Can you work these out from the model? Positions are in its coordinate system, mm. Face numbers are marked on the shaded views. A direction names the side the tool comes from. Coordinates: 2 decimals unless noted, no trailing zeros. Order: outer loops, then holes, each group sorted by start corner. A loop starts at its lowest first (then second) coordinate and runs counter-clockwise, first axis right, second up. Notation, with made-up numbers: (-35.75, 19) - (22.25, 19) arc R19 cw to (22.25, 55) - close; hole circle Ø2 at (-36, 30). An arc over 180 degrees is marked (long way). Use a Markdown table: item, result. Add a question column.
(1) I want a section at D-D (x = -130). List the corners of the cut face in (y, z) for me.
(2) On a 3-axis mill with a long thin cutter (end or side, diameter ignored), from which of +Z, -Z, +X, -X, +Y, -Y can I reach the whole of each face in a straight line? I mean the marked faces 1, 2, 3 and 4. Say none if no direction works.
(3) I want a section at C-C (z = 35.5). List the corners of the cut face in (x, y) for me.
(4) I want a section at A-A (z = 126). List the corners of the cut face in (x, y) for me, and give its area (3 significant figures).
(5) We'd pull the mould along X, two halves only. Please class the marked faces 5, 6 and 7: pulls with the +X half, pulls with the -X half, needs draft (parallel to the pull), parting line crosses it, or undercut.
(6) I want a section at B-B (y = -60). List the corners of the cut face in (x, z) for me.
(7) If I drill on L1, parallel to X at y = -6, z = 99.5; L2, parallel to X at y = -62.5, z = -63.5; L3, parallel to Z at x = 231, y = -20, over which ranges is the centre line in solid material (lowest first)? Write a range as [from, to].
(8) For pin 1 Ø12 at (y, z) = (-14, -99.5) entering from -X; pin 2 Ø21 at (x, y) = (171.5, -45.5) entering from +Z; pin 3 Ø10 at (y, z) = (-28.5, 178) entering from +X, each with a flat end and sliding along its axis, tell me the tip position at first contact or that it passes through.
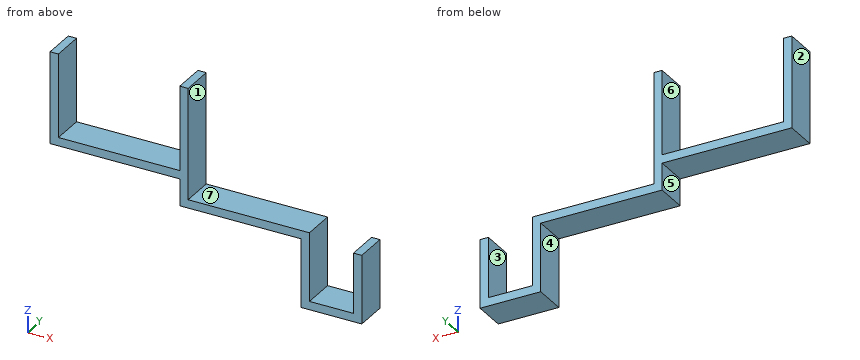
```python
from build123d import *

# Parameters (mm, degrees)
F0_W     = 18
F0_H     = 18
F0_H_2   = 130
F0_H_3   = 180
F1_DEPTH = 70


with BuildPart() as f1:
    # F0 (on Front) → F1 (new body)
    with BuildSketch(Plane.XZ):
        with Locations((-9, 9)):
            Rectangle(F0_W, F0_H)
        Polygon((0, 18), (0, 0), (244, 0), (262, 0), (262, 18), align=None)
        Polygon((-18, 18), (0, 18), (0, 258), (-18, 258), (-18, 76), (-18, 66.81706), (-18, 58), align=None)
        with Locations((253, -65)):
            Rectangle(F0_W, F0_H_2)
        Polygon((262, -130), (244, -130), (244, -148), (357, -148), (357, -130), align=None)
        Polygon((-298, 58), (-18, 58), (-18, 66.81706), (-18, 76), (-280, 76), (-298, 76), align=None)
        with Locations((366, -65)):
            Rectangle(F0_W, F0_H_2)
        with Locations((366, -139)):
            Rectangle(F0_W, F0_H)
        with Locations((-289, 166)):
            Rectangle(F0_W, F0_H_3)
    extrude(amount=F1_DEPTH)


solid = f1.part
```
Answers follow:
| question | item | result |
|---|---|---|
| 1 | outline | (-70, 58) - (0, 58) - (0, 76) - (-70, 76) - close |
| 2 | face 1 | +Z, +X, +Y, -Y |
| 2 | face 2 | +Z, -Z, -X, +Y, -Y |
| 2 | face 3 | +Z, +Y, -Y |
| 2 | face 4 | -Z, -X, +Y, -Y |
| 3 | outline | (-18, -70) - (0, -70) - (0, 0) - (-18, 0) - close |
| 4 | outline | (-298, -70) - (-280, -70) - (-280, 0) - (-298, 0) - close; (-18, -70) - (0, -70) - (0, 0) - (-18, 0) - close |
| 4 | area | 2,520 mm² |
| 5 | face 5 | pulls with the -X half |
| 5 | face 6 | undercut |
| 5 | face 7 | needs draft |
| 6 | outline | (-298, 58) - (-18, 58) - (-18, 0) - (244, 0) - (244, -148) - (375, -148) - (375, 0) - (357, 0) - (357, -130) - (262, -130) - (262, 18) - (0, 18) - (0, 258) - (-18, 258) - (-18, 76) - (-280, 76) - (-280, 256) - (-298, 256) - close |
| 7 | L1 | x = [-298, -280], [-18, 0] |
| 7 | L2 | x = [244, 262], [357, 375] |
| 7 | L3 | z = [0, 18] |
| 8 | pin 1 | stops at x = 244 |
| 8 | pin 2 | stops at z = 18 |
| 8 | pin 3 | stops at x = 0 |
